```python
from build123d import *

# Parameters (mm, degrees)
F0_R     = 55
F0_R_2   = 2.75
F0_R_3   = 2
F0_R_4   = 5
F1_DEPTH = 2
F2_SIZE2 = 1
F2_SIZE  = 8.5
F3_SIZE2 = 8
F3_SIZE  = 1


with BuildPart() as f1:
    # F0 (on Top) → F1 (new body)
    with BuildSketch(Plane.XY):
        Circle(F0_R)
        with Locations((0, -37)):
            Circle(F0_R_2, mode=Mode.SUBTRACT)
        with Locations((26.5, -25.5)):
            Circle(F0_R_3, mode=Mode.SUBTRACT)
        with Locations((26.5, 0)):
            Circle(F0_R_4, mode=Mode.SUBTRACT)
        with Locations((26.5, 25.5)):
            Circle(F0_R_3, mode=Mode.SUBTRACT)
        with Locations((0, 37)):
            Circle(F0_R_2, mode=Mode.SUBTRACT)
    extrude(amount=F1_DEPTH)

    # F2
    f2_edges = [f1.edges().sort_by_distance(p)[0] for p in [
        (-55, 0, 2),
    ]]
    f2_side = f1.faces().sort_by_distance((-0.293764, 0, 2))[0]
    chamfer(f2_edges, length=F2_SIZE, length2=F2_SIZE2, reference=f2_side)

    # F3
    f3_edges = [f1.edges().sort_by_distance(p)[0] for p in [
        (21.5, 0, 2),
    ]]
    f3_side = f1.faces().sort_by_distance((21.5, 0, 1))[0]
    chamfer(f3_edges, length=F3_SIZE, length2=F3_SIZE2, reference=f3_side)


solid = f1.part
```
For this review, take the finished solid that the model builds, in its own axes (mm). Give positions to 0.01 mm unless a question says otherwise; leave off trailing zeros. Write each loop counter-clockwise with the first axis right and the second up, starting at its lowest first coordinate (ties: lowest second). Pieces come first, ordered by that corner, then holes. Notation, with made-up numbers: M 69.5,-9.5 L 81.5,-9.5 A25 ccw 81.5,6.5 Z; hole C 58.5,6 d5. An arc over 180 degrees is marked long. One line per item, written item: value.
1) For line 1 (Y direction, x = 0, z = 0.6); line 2 (Y direction, x = 26.5, z = 0.65); line 3 (X direction, y = 13, z = 0.6), list the stretches that pass through material, from the lowest coordinate up. Write a range as from..to.
Results are:
line 1: y = -55..-39.75, -34.25..34.25, 39.75..55
line 2: y = -48.19..-27.5, -23.5..-5, 5..23.5, 27.5..48.19
line 3: x = -53.44..53.44
2) Take a section at C-C, the plane x = 27. Count the separate pieces of the cut face and the enclosed holes in it, then the cut area to 3 significant figures.
Results are:
separate pieces: 4
enclosed holes: 0
area: 138 mm²
3) The part is to be moulded in two halves that separate along X. For faces 1 (the cylindrical face through (-0.358, -34.273, 0.986)), 2 (the flat face through (-1, 1, 2)), 3 (the cylindrical face through (-11.923, -53.692, 0.493)), say which applies: +X half, -X half, draft (parallel to the pull), parting line (faces both ways), or undercut.
Results are:
face 1: undercut
face 2: draft
face 3: parting line
4) Take a section at A-A, the plane x = 0. Write out the cut boundary in (y, z).
Results are:
outline: M -55,0 L -39.75,0 L -39.75,2 L -46.5,2 L -55,1 Z; M -34.25,0 L 34.25,0 L 34.25,2 L -34.25,2 Z; M 39.75,0 L 55,0 L 55,1 L 46.5,2 L 39.75,2 Z
5) Take a section at B-B, the plane z = 0.4. Write out the cut boundary in (x, y), then the cut area to 3 significant figures.
Results are:
outline: C 0,0 d110; hole C 0,-37 d5.5; hole C 0,37 d5.5; hole C 26.5,0 d10; hole C 26.5,-25.5 d4; hole C 26.5,25.5 d4
area: 9,350 mm²
